```python
from build123d import *

# Parameters (mm, degrees)
F1_DEPTH = 21.1
F3_DEPTH = 22
F5_DEPTH = 25
F6_R     = 3.15
F7_DEPTH = 2.5
F8_R     = 3.15
F9_DEPTH = 2
F10_R    = 5
F11_R    = 5
F12_R    = 5


with BuildPart() as f1:
    # F0 (on Top) → F1 (new body)
    with BuildSketch(Plane.XY):
        with BuildLine():
            ThreePointArc((-22, 0), (-28, -6), (-34, 0))
            Line((-34, 0), (-37, 0))
            ThreePointArc((-37, 0), (-28.7526363425, -8.9684747051), (-19.1258803254, -1.5))
            Line((-19.1258803254, -1.5), (19.1258803254, -1.5))
            ThreePointArc((19.1258803254, -1.5), (28.7526363425, -8.9684747051), (37, 0))
            Line((37, 0), (34, 0))
            ThreePointArc((34, 0), (28, -6), (22, 0))
            Line((22, 0), (22, 1.5))
            Line((22, 1.5), (-22, 1.5))
            Line((-22, 1.5), (-22, 0))
        make_face()
    extrude(amount=F1_DEPTH)

    # F2 (on face) → F3 (join)
    with BuildSketch(Plane.XY.offset(21.1)):
        Polygon((-22, 0), (-22, -1.5), (-19.1258803254, -1.5), (19.1258803254, -1.5), (22, -1.5), (22, 0), (22, 1.5), (-22, 1.5), align=None)
    extrude(amount=F3_DEPTH)

    # F4 (on face) → F5 (join)
    with BuildSketch(Plane.XY.offset(43.1)):
        with BuildLine():
            ThreePointArc((-34, 0), (-28, 6), (-22, 0))
            Line((-22, 0), (-22, -1.5))
            Line((-22, -1.5), (22, -1.5))
            Line((22, -1.5), (22, 0))
            ThreePointArc((22, 0), (28, 6), (34, 0))
            Line((34, 0), (37, 0))
            ThreePointArc((37, 0), (28.7526363425, 8.9684747051), (19.1258803254, 1.5))
            Line((19.1258803254, 1.5), (-19.1258803254, 1.5))
            ThreePointArc((-19.1258803254, 1.5), (-28.7526363425, 8.9684747051), (-37, 0))
            Line((-37, 0), (-34, 0))
        make_face()
    extrude(amount=F5_DEPTH)

    # F6 (on Right) → F7 (join, symmetric)
    with BuildSketch(Plane.YZ):
        with BuildLine():
            Line((0, 68.1), (-26.5, 68.1))
            ThreePointArc((-26.5, 68.1), (-35.7387953251, 61.9268343237), (-33.5710678119, 51.0289321881))
            Line((-33.5710678119, 51.0289321881), (0, 17.4578643763))
            Line((0, 17.4578643763), (0, 68.1))
        make_face()
        with Locations((-26.5, 58.1)):
            Circle(F6_R, mode=Mode.SUBTRACT)
    extrude(amount=F7_DEPTH, both=True)

    # F8 (on face) → F9 (cut)
    with BuildSketch(Plane(origin=(-2.5, 0, 0), x_dir=(0, -1, 0), z_dir=(-1, 0, 0))):
        Polygon((31.65, 61.0733538863), (26.5, 64.0467077727), (21.35, 61.0733538863), (21.35, 55.1266461137), (26.5, 52.1532922273), (31.65, 55.1266461137), align=None)
        with Locations((26.5, 58.1)):
            Circle(F8_R, mode=Mode.SUBTRACT)
    extrude(amount=-F9_DEPTH, mode=Mode.SUBTRACT)

    # F10
    f10_edges = [f1.edges().sort_by_distance(p)[0] for p in [
        (-2.5, -1.5, 43.528932),
        (2.5, -1.5, 43.528932),
    ]]
    fillet(f10_edges, radius=F10_R)

    # F11
    f11_edges = [f1.edges().sort_by_distance(p)[0] for p in [
        (0, -1.5, 18.957864),
    ]]
    fillet(f11_edges, radius=F11_R)

    # F12
    f12_edges = [f1.edges().sort_by_distance(p)[0] for p in [
        (-19.12588, -1.5, 10.55),
        (19.12588, -1.5, 10.55),
        (-19.12588, 1.5, 55.6),
        (19.12588, 1.5, 55.6),
    ]]
    fillet(f12_edges, radius=F12_R)


solid = f1.part
```
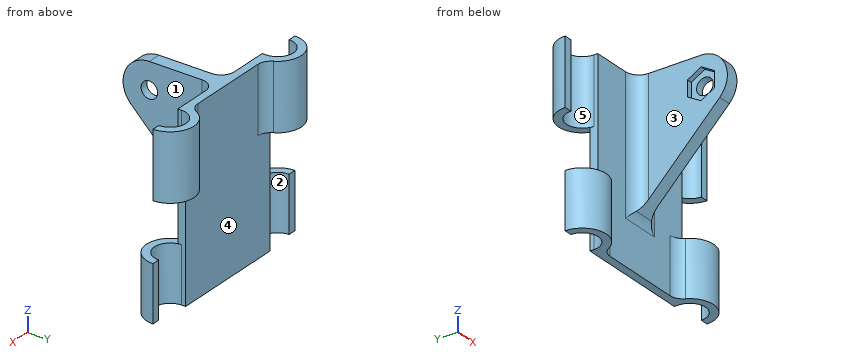
Work out the finished part from the listing and answer in its coordinate system (mm). Face numbers are marked on the shaded views. A direction names the side the tool comes from. Round coordinates to 2 decimals unless told otherwise and drop trailing zeros. Write each loop counter-clockwise with the first axis right and the second up, starting at its lowest first coordinate (ties: lowest second). Pieces come first, ordered by that corner, then holes. Notation, with made-up numbers: (-6.5, 45.25) - (1.5, 45.25) arc R25 ccw to (1.5, 82.25) - close; hole circle Ø11 at (-38, 47). An arc over 180 degrees is marked (long way). Return JSON: item names as keys, results as strings. Group by question number.
Q1. For the marked faces 4 and 5, determine the directions among +Z, -Z, +X, -X, +Y, -Y from which every point of the face is accessible in a straight line to the end or side of a thin tool.
Q2. The part is cut by section A-A on z = 58.1. Write down the section's boundary in (x, y).
Q3. The part is cut by section D-D on x = 11. Write down the section's boundary in (y, z).
Q4. Find the intervals of material crossed by L1, parallel to Y at x = 1.45, z = 58.1; L2, parallel to Y at x = 21, z = 28.5; L3, parallel to Z at x = 0, y = -26, in increasing order.
Q5. The part is cut by section C-C on z = 5. Write down the section's boundary in (x, y).
Q6. Each of these flat-tipped pins is pushed along its axis until it touches: pin 1 Ø6 at (y, z) = (0, 35.5) entering from +X; pin 2 Ø4 at (y, z) = (-24, 57) entering from -X; pin 3 Ø5 at (y, z) = (-4.5, 37.5) entering from -X; pin 4 Ø2 at (x, z) = (-2, 59) entering from -Y. Where does it stop, or does it pass through?
Q7. The mould has two halves that part along X. Classify the marked faces 1, 2 and 3: released by +X, released by -X, zero draft, split by the parting line, or undercut.
Q8. The part is cut by section B-B on x = 28. Write down the section's boundary in (y, z).
Solved:
{
 "1": {"face 4": "-Z, +Y", "face 5": "+Z, -Z, -Y"},
 "2": {"outline": "(-37, 0) - (-34, 0) arc R6 cw to (-22, 0) - (-22, -1.5) - (-7.5, -1.5) arc R5 cw to (-2.5, -6.5) - (-2.5, -21.35) - (-0.5, -21.35) - (-0.5, -23.35) - (2.5, -23.35) - (2.5, -6.5) arc R5 cw to (7.5, -1.5) - (22, -1.5) - (22, 0) arc R6 cw to (34, 0) - (37, 0) arc R9 ccw to (20.03, 4.18) arc R5 cw to (15.6, 1.5) - (-15.6, 1.5) arc R5 cw to (-20.03, 4.18) arc R9 ccw to start; (-2.5, -36.5) - (2.5, -36.5) - (2.5, -29.65) - (-0.5, -29.65) - (-0.5, -31.65) - (-2.5, -31.65) - close"},
 "3": {"outline": "(-1.5, 0) - (1.5, 0) - (1.5, 68.1) - (-1.5, 68.1) - close"},
 "4": {"L1": "-36.5 to -29.65, -23.35 to 1.5", "L2": "-1.5 to 1.5", "L3": "43.46 to 54.99, 61.21 to 68.1"},
 "5": {"outline": "(-37, 0) arc R9 ccw to (-20.03, -4.18) arc R5 cw to (-15.6, -1.5) - (15.6, -1.5) arc R5 cw to (20.03, -4.18) arc R9 ccw to (37, 0) - (34, 0) arc R6 cw to (22, 0) - (22, 1.5) - (-22, 1.5) - (-22, 0) arc R6 cw to (-34, 0) - close"},
 "6": {"pin 1": "x = 22", "pin 2": "x = -0.5", "pin 3": "x = -5.32", "pin 4": "y = -36.5"},
 "7": {"face 1": "released by +X", "face 2": "undercut", "face 3": "released by -X"},
 "8": {"outline": "(-9, 0) - (-6, 0) - (-6, 21.1) - (-9, 21.1) - close; (6, 43.1) - (9, 43.1) - (9, 68.1) - (6, 68.1) - close"}
}
